```python
from build123d import *

# Parameters (mm, degrees)
SKETCH_W        = 65
SKETCH_H        = 20
PAD_DEPTH       = 5
SKETCH001_W     = 31.226576
SKETCH001_H     = 20
SKETCH001_W_2   = 5.773424
PAD001_DEPTH    = 8
POCKET_DEPTH    = 31.226576
PAD002_DEPTH    = 25
SKETCH003_R     = 1
POCKET001_DEPTH = 20.001


with BuildPart() as pocket001:
    # Sketch → Pad (new body)
    with BuildSketch(Plane.XY):
        with Locations((2.5, 0)):
            Rectangle(SKETCH_W, SKETCH_H)
    extrude(amount=PAD_DEPTH)

    # Sketch001 → Pad001 (new body)
    with BuildSketch(Plane.XY.offset(5)):
        with Locations((19.386712, 0)):
            Rectangle(SKETCH001_W, SKETCH001_H)
        with Locations((-27.113288, 0)):
            Rectangle(SKETCH001_W_2, SKETCH001_H)
    extrude(amount=PAD001_DEPTH)

    # Sketch002 → Pocket (cut)
    with BuildSketch(Plane.YZ.offset(35)):
        with BuildLine():
            Line((-2.73443, 15), (-2.73443, 6.487833))
            ThreePointArc((-2.73443, 6.487833), (0, 3.753403), (2.73443, 6.487833))
            Line((2.73443, 15), (2.73443, 6.487833))
            Line((-2.73443, 15), (2.73443, 15))
        make_face()
    extrude(amount=-POCKET_DEPTH, mode=Mode.SUBTRACT)

    # Sketch004 → Pad002 (new body)
    with BuildSketch(Plane.XY.offset(13)):
        with BuildLine():
            ThreePointArc((26.060559, -2.73443), (22.427774, -6.367215), (26.060559, -10))
            Line((26.060559, -10), (31.367215, -10))
            ThreePointArc((31.367215, -10), (35, -6.367215), (31.367215, -2.73443))
            Line((26.060559, -2.73443), (31.367215, -2.73443))
        make_face()
    extrude(amount=PAD002_DEPTH)

    # Sketch003 → Pocket001 (cut, through all)
    with BuildSketch(Plane.XZ.offset(10)):
        with Locations((28, 35)):
            Circle(SKETCH003_R)
    extrude(amount=-POCKET001_DEPTH, mode=Mode.SUBTRACT)


with BuildPart() as part_mirroring:
    # Part__Mirroring: instance of Pocket001
    add(pocket001.part.mirror(Plane(origin=(0, 0, 0), x_dir=(1, 0, 0), z_dir=(0, 1, 0))))


with BuildPart() as fusion:
    # Fusion base: copy of Pocket001
    add(pocket001.part)

    # Fusion: union Part__Mirroring
    add(part_mirroring.part)


solid = fusion.part
```
Source: CAD feature listing. Evaluate the final solid. Frame: model axes, mm. A direction names the side the tool comes from. Give positions to 0.01 mm unless a question says otherwise; leave off trailing zeros. Loops run counter-clockwise (first coordinate to the right, second up) from the corner with the lowest first, then second, coordinate; pieces in that order, holes last. Notation, with made-up numbers: (88, -37) -> (113, -37) arc R30 ccw to (113, -1) -> close; hole circle Ø3 at (84.5, 11). An arc over 180 degrees is marked (long way). Put each result on its own line as item: value. Start each with the question number.
1) Material intervals for probe 1 along Y at (x, z) = (7, 9); probe 2 along Z at (x, y) = (28, 4.5); probe 3 along X at (y, z) = (3.25, 8), sorted ascending.
2) Reachability of faces 4 (the face through (22.43, 6.29, 25.32)), 5 (the face through (3.773, 0, 4.5)), 6 (the face through (-24.227, 0, 9)) from +Z, -Z, +X, -X, +Y, -Y: full face, straight path, thin tool, end or side. Return the list, or none.
3) Cut plane C-C (z = 32). Return loops of the section in (x, y), then the cut area to 3 significant figures.
4) Cut plane B-B (z = 10.5). Return loops of the section in (x, y).
5) Contact query for flat-ended pins moving along their axis: P1, Ø2, axis at x = 16, y = -7.5, coming from the +Z side; P2, Ø12, axis at x = -3.5, z = 20.5, coming from the -Y side; P3, Ø1.8, axis at x = 34, y = 9, coming from the +Z side; P4, Ø1, axis at x = -2, y = -1, coming from the +Z side. Output: stop coordinate, or through.
6) Draft query along Y for faces 1 (the face through (23, 2.734, 12)), 2 (the face through (-27, 0, 13)), 3 (the face through (12, 10, 9)). Return one class per face: released by +Y, released by -Y, zero draft, split by the parting line, or undercut.
7) Cut plane D-D (y = 0). Return loops of the section in (x, z), then the cut area to 3 significant figures.
8) Cut plane A-A (x = 28). Return loops of the section in (y, z).
Results are:
1. probe 1: y = -10 to -2.73, 2.73 to 10
1. probe 2: z = 0 to 34, 36 to 38
1. probe 3: x = -30 to -24.23, 3.77 to 35
2. face 4: +Z, -X
2. face 5: +Z, +X
2. face 6: +Z, +Y, -Y
3. outline: (26.06, -10) -> (31.37, -10) arc R3.63 ccw to (31.37, -2.73) -> (26.06, -2.73) arc R3.63 ccw to start; (26.06, 2.73) -> (31.37, 2.73) arc R3.63 ccw to (31.37, 10) -> (26.06, 10) arc R3.63 ccw to start
3. area: 160 mm2
4. outline: (-30, -10) -> (-24.23, -10) -> (-24.23, 10) -> (-30, 10) -> close; (3.77, -10) -> (35, -10) -> (35, -2.73) -> (3.77, -2.73) -> close; (3.77, 2.73) -> (35, 2.73) -> (35, 10) -> (3.77, 10) -> close
5. P1: stops at z = 13
5. P2: passes through
5. P3: stops at z = 38
5. P4: stops at z = 5
6. face 1: undercut
6. face 2: zero draft
6. face 3: released by +Y
7. outline: (-30, 0) -> (35, 0) -> (35, 3.75) -> (3.77, 3.75) -> (3.77, 5) -> (-24.23, 5) -> (-24.23, 13) -> (-30, 13) -> close
7. area: 332 mm2
8. outline: (-10, 0) -> (10, 0) -> (10, 34) -> (2.73, 34) -> (2.73, 6.49) arc R2.73 cw to (-2.73, 6.49) -> (-2.73, 34) -> (-10, 34) -> close; (-10, 36) -> (-2.73, 36) -> (-2.73, 38) -> (-10, 38) -> close; (2.73, 36) -> (10, 36) -> (10, 38) -> (2.73, 38) -> close
